Verification items for the finished model (mm, model axes). A direction names the side the tool comes from. Give positions to 0.01 mm unless a question says otherwise; leave off trailing zeros. Order: outer loops, then holes, each group sorted by start corner. A loop starts at its lowest first (then second) coordinate and runs counter-clockwise, first axis right, second up.
from build123d import *

# Parameters (mm, degrees)
SKETCH_W                = 100
SKETCH_H                = 60
PAD_DEPTH               = 10
THICKNESS_T             = -2
SKETCH001_R             = 2
PAD001_DEPTH            = 2
SKETCH001_MIRRORED_2_R  = 2
PAD001_MIRRORED_2_DEPTH = 2


with BuildPart() as part:
    # Sketch → Pad (new body)
    with BuildSketch(Plane.XY):
        Rectangle(SKETCH_W, SKETCH_H)
    extrude(amount=PAD_DEPTH)

    # Thickness
    thickness_openings = [part.faces().sort_by_distance(p)[0] for p in [
        (0, 0, 10),
    ]]
    offset(amount=THICKNESS_T, openings=thickness_openings)

    # Sketch001 (on Face6 of Thickness) → Pad001 (join)
    with BuildSketch(Plane.XY.offset(10)):
        with BuildLine():
            Line((-61, -9.292408), (-48, -9.292408))
            Line((-48, -9.292408), (-48, -20.993994))
            Line((-48, -20.993994), (-61, -20.993994))
            ThreePointArc((-63, -18.993994), (-62.414214, -20.408207), (-61, -20.993994))
            Line((-63, -18.993994), (-63, -11.292408))
            ThreePointArc((-61, -9.292408), (-62.414214, -9.878194), (-63, -11.292408))
        make_face()
        with Locations((-58, -15.143201)):
            Circle(SKETCH001_R, mode=Mode.SUBTRACT)
    pad001 = extrude(amount=-PAD001_DEPTH)

    # Sketch001 Mirrored 2 → Pad001 Mirrored 2 (add)
    with BuildSketch(Plane(origin=(0, 0, 10), x_dir=(-1, 0, 0), z_dir=(0, 0, -1))):
        with BuildLine():
            Line((-61, -9.292408), (-48, -9.292408))
            Line((-48, -9.292408), (-48, -20.993994))
            Line((-48, -20.993994), (-61, -20.993994))
            ThreePointArc((-63, -18.993994), (-62.414214, -20.408207), (-61, -20.993994))
            Line((-63, -18.993994), (-63, -11.292408))
            ThreePointArc((-61, -9.292408), (-62.414214, -9.878194), (-63, -11.292408))
        make_face()
        with Locations((-58, -15.143201)):
            Circle(SKETCH001_MIRRORED_2_R, mode=Mode.SUBTRACT)
    pad001_mirrored_2 = extrude(amount=PAD001_MIRRORED_2_DEPTH)

    # Mirrored001: Pad001, Pad001 Mirrored 2 across XZ
    add(pad001.mirror(Plane.XZ))
    add(pad001_mirrored_2.mirror(Plane.XZ))


solid = part.part
(1) Section check D-D, the plane x = -13.5. Enter the section's corners in (y, z).
Solved:
outline: (-30, 0) - (30, 0) - (30, 10) - (28, 10) - (28, 2) - (-28, 2) - (-28, 10) - (-30, 10) - close
(2) Go/stop test with flat-tipped pins: pin 1 (12 mm diameter, centred on x = 16, y = -11, fed in from +Z); pin 2 (1 mm diameter, centred on y = 5, z = 2.5, fed in from +X); pin 3 (0.6 mm diameter, centred on x = 54.5, z = 9.5, fed in from -Y). Record where each tip stops, or that it passes through.
Solved:
pin 1: stops at z = 2
pin 2: stops at x = 50
pin 3: stops at y = -20.99
(3) Section check A-A, the plane z = 5.25. Enter the section's corners in (x, y), then the cut area to 3 significant figures.
Solved:
outline: (-50, -30) - (50, -30) - (50, 30) - (-50, 30) - close; hole (-48, -28) - (48, -28) - (48, 28) - (-48, 28) - close
area: 624 mm2
(4) Set-up check for faces 4 (the flat face through (48, 0, 6)), 5 (the flat face through (55, -15, 8)), 6 (the flat face through (-1, -30, 5)), 7 (the flat face through (-55, -15, 8)), 8 (the cylindrical face through (-56.092, 14.542, 9.014)): record each of +Z, -Z, +X, -X, +Y, -Y from which the full face is reachable in a straight line by a thin tool's end or side.
Solved:
face 4: +Z
face 5: -Z, +X, +Y, -Y
face 6: +Z, -Z, +X, -X, -Y
face 7: -Z, -X, +Y, -Y
face 8: +Z, -Z
(5) Scan lines: line 1 (Y direction, x = -58, z = 9.6); line 2 (X direction, y = -15, z = 3.25); line 3 (Y direction, x = -8.5, z = 4). Record each from-to range of solid material in increasing order.
Solved:
line 1: y = -20.99 to -17.14, -13.14 to -9.29, 9.29 to 13.14, 17.14 to 20.99
line 2: x = -50 to -48, 48 to 50
line 3: y = -30 to -28, 28 to 30
(6) Section check C-C, the plane y = -8. Enter the section's corners in (x, z).
Solved:
outline: (-50, 0) - (50, 0) - (50, 10) - (48, 10) - (48, 2) - (-48, 2) - (-48, 10) - (-50, 10) - close
(7) Section check B-B, the plane x = 58. Enter the section's corners in (y, z), then the cut area to 3 significant figures.
Solved:
outline: (-20.99, 8) - (-17.14, 8) - (-17.14, 10) - (-20.99, 10) - close; (-13.14, 8) - (-9.29, 8) - (-9.29, 10) - (-13.14, 10) - close; (9.29, 8) - (13.14, 8) - (13.14, 10) - (9.29, 10) - close; (17.14, 8) - (20.99, 8) - (20.99, 10) - (17.14, 10) - close
area: 30.8 mm2
(8) Release check for a two-part mould opening along Y. For faces 1 (the flat face through (-1, 0, 0)), 2 (the flat face through (-1, 0, 2)), 3 (the flat face through (-1, 30, 5)) record: pulls with the +Y half, pulls with the -Y half, needs draft (parallel to the pull), parting line crosses it, or undercut.
Solved:
face 1: needs draft
face 2: undercut
face 3: pulls with the +Y half
